```python
from build123d import *

# Parameters (mm, degrees)
SKETCH1_R                      = 16.5
BOSS_EXTRUDE1_DEPTH            = 3
CBORE_FOR_M2_SHCS1_D           = 2.4
CBORE_FOR_M2_SHCS1_CBORE_D     = 4.4
CBORE_FOR_M2_SHCS1_CBORE_DEPTH = 2
CIRPATTERN1_COUNT              = 4
SKETCH8_R                      = 0.5
CUT_EXTRUDE1_DEPTH             = 1.5


with BuildPart() as part:
    # Sketch1 → Boss-Extrude1 (new body)
    with BuildSketch(Plane(origin=(0, 0, 0), x_dir=(1, 0, 0), z_dir=(0, 1, 0))):
        with Locations(Location((0, 0, 0), (0, 0, 270))):
            Circle(SKETCH1_R)
    extrude(amount=BOSS_EXTRUDE1_DEPTH)

    # CBORE for M2 SHCS1 (through all)
    with Locations(Plane(origin=(0, 3, 0), x_dir=(1, 0, 0), z_dir=(0, 1, 0))):
        with Locations((13, 0)):
            cbore_for_m2_shcs1 = CounterBoreHole(CBORE_FOR_M2_SHCS1_D / 2, CBORE_FOR_M2_SHCS1_CBORE_D / 2, CBORE_FOR_M2_SHCS1_CBORE_DEPTH)

    # CirPattern1: CBORE for M2 SHCS1 ×4 about axis
    cirpattern1_axis = Axis((0, 0, 0), (0, 1, 0))
    for i in range(1, CIRPATTERN1_COUNT):
        add(cbore_for_m2_shcs1.rotate(cirpattern1_axis, i * 360 / CIRPATTERN1_COUNT), mode=Mode.SUBTRACT)

    # Sketch8 → Cut-Extrude1 (cut)
    with BuildSketch(Plane.XZ):
        with Locations(Location((6, 0, 0), (0, 0, 270))):
            Circle(SKETCH8_R)
    extrude(amount=-CUT_EXTRUDE1_DEPTH, mode=Mode.SUBTRACT)


solid = part.part
```
Model file for the job. Use its own axes, mm. A direction names the side the tool comes from. Coordinates: 2 decimals unless noted, no trailing zeros. Order: outer loops, then holes, each group sorted by start corner. A loop starts at its lowest first (then second) coordinate and runs counter-clockwise, first axis right, second up. Notation, with made-up numbers: (-28, -22.75) - (-11, -22.75) arc R19 cw to (-11, 14.25) - close; hole circle Ø1 at (84, -10). An arc over 180 degrees is marked (long way). Return JSON: item names as keys, results as strings. Group by question number.
1) Saw through at C-C, the plane x = -13. Write the cut outline in (y, z).
2) Saw through at A-A, the plane z = 0. Write the cut outline in (x, y).
3) Probe line 1 (Z direction, x = -14, y = 2.7); line 2 (X direction, y = 2.45, z = -12.5); line 3 (Z direction, x = -13, y = 0.55). List the from-to ranges inside material, lowest first. Write a range as from..to.
4) Saw through at D-D, the plane x = -0.5. Write the cut outline in (y, z), plus the area to 3 significant figures.
5) Mould opens along Z. For faces 4 (the cylindrical face through (-16.108, 1.479, -3.577)), 5 (the cylindrical face through (15.032, 2.014, 0.843)), 6 (the flat face through (0, 3, 0)) say: released by +Z, released by -Z, zero draft, split by the parting line, or undercut.
6) Saw through at B-B, the plane z = -13. Write the cut outline in (x, y), plus the area to 3 significant figures.
7) Tool access for faces 1 (the cylindrical face through (-0.843, 2.014, 15.032)), 2 (the cylindrical face through (-11.855, 0.493, 0.36)), 3 (the flat face through (6, 1.5, 0)): list every direction of +Z, -Z, +X, -X, +Y, -Y with a clear straight run to the whole face (end or side of a thin tool).
8) Flat gauge pins, fed straight in: P1, Ø1.4, axis at x = 13, z = 0, coming from the -Y side; P2, Ø10, axis at x = 0.5, z = 1, coming from the -Y side; P3, Ø1.5, axis at y = 2, z = 7, coming from the +X side; P4, Ø4, axis at x = 0, z = 13, coming from the +Y side. Where does each tip first touch, or does it go through?
Values found:
{
 "1": {"outline": "(0, -10.16) - (3, -10.16) - (3, -2.2) - (1, -2.2) - (1, -1.2) - (0, -1.2) - close; (0, 1.2) - (1, 1.2) - (1, 2.2) - (3, 2.2) - (3, 10.16) - (0, 10.16) - close"},
 "2": {"outline": "(-16.5, 0) - (-14.2, 0) - (-14.2, 1) - (-15.2, 1) - (-15.2, 3) - (-16.5, 3) - close; (-11.8, 0) - (5.5, 0) - (5.5, 1.5) - (6.5, 1.5) - (6.5, 0) - (11.8, 0) - (11.8, 1) - (10.8, 1) - (10.8, 3) - (-10.8, 3) - (-10.8, 1) - (-11.8, 1) - close; (14.2, 0) - (16.5, 0) - (16.5, 3) - (15.2, 3) - (15.2, 1) - (14.2, 1) - close"},
 "3": {"line 1": "z = -8.73..-1.96, 1.96..8.73", "line 2": "x = -10.77..-2.14, 2.14..10.77", "line 3": "z = -10.16..-1.2, 1.2..10.16"},
 "4": {"outline": "(0, -16.49) - (3, -16.49) - (3, -15.14) - (1, -15.14) - (1, -14.09) - (0, -14.09) - close; (0, -11.91) - (1, -11.91) - (1, -10.86) - (3, -10.86) - (3, 10.86) - (1, 10.86) - (1, 11.91) - (0, 11.91) - close; (0, 14.09) - (1, 14.09) - (1, 15.14) - (3, 15.14) - (3, 16.49) - (0, 16.49) - close", "area": "77.5 mm²"},
 "5": {"face 4": "split by the parting line", "face 5": "undercut", "face 6": "zero draft"},
 "6": {"outline": "(-10.16, 0) - (-1.2, 0) - (-1.2, 1) - (-2.2, 1) - (-2.2, 3) - (-10.16, 3) - close; (1.2, 0) - (10.16, 0) - (10.16, 3) - (2.2, 3) - (2.2, 1) - (1.2, 1) - close", "area": "49.8 mm²"},
 "7": {"face 1": "+Y", "face 2": "+Y, -Y", "face 3": "-Y"},
 "8": {"P1": "passes through", "P2": "stops at y = 0", "P3": "stops at x = 15.27", "P4": "stops at y = 1"}
}
